Check sheet for the drawn part. Datum: minimum x, y, z corner. Units: mm. A direction names the side the tool comes from. Coordinates: 2 decimals unless noted, no trailing zeros. Order: outer loops, then holes, each group sorted by start corner. A loop starts at its lowest first (then second) coordinate and runs counter-clockwise, first axis right, second up. Notation, with made-up numbers: M -23,58.5 L -18,58.5 A13 cw -18,64.5 Z; hole C 85,-16 d7. An arc over 180 degrees is marked long. Return JSON: item names as keys, results as strings. Group by question number.
Q1. Section check A-A, the plane z = 24.5. Enter the section's corners in (x, y).
Q2. Section check C-C, the plane y = 24. Enter the section's corners in (x, z).
Q3. Mould release check, pull along Y, two halves, no side actions. Record for the marked faces 3, 4, 5 and 6: pulls with the +Y half, pulls with the -Y half, needs draft (parallel to the pull), parting line crosses it, or undercut.
Q4. Section check B-B, the plane x = 180. Enter the section's corners in (y, z), then the cut area to 3 significant figures.
Q5. Thickness scan on probe 1 along Y at (x, z) = (5, 22.5); probe 2 along X at (y, z) = (130.2, 18.25); probe 3 along X at (y, z) = (123.5, 24.75). Record the ranges inside material, lowest first.
Q6. Access from +Z, -Z, +X, -X, +Y, -Y to the whole of each face (thin tool, end or side, straight path). Record for the marked faces 1 and 2.
Q7. Section check D-D, the plane x = 37. Enter the section's corners in (y, z).
Q8. Go/stop test with flat-tipped pins: pin 1 Ø0.9 at (x, y) = (208.5, 5) entering from +Z; pin 2 Ø2.5 at (x, y) = (155.5, 89.5) entering from +Z. Record where each tip stops, or that it passes through.
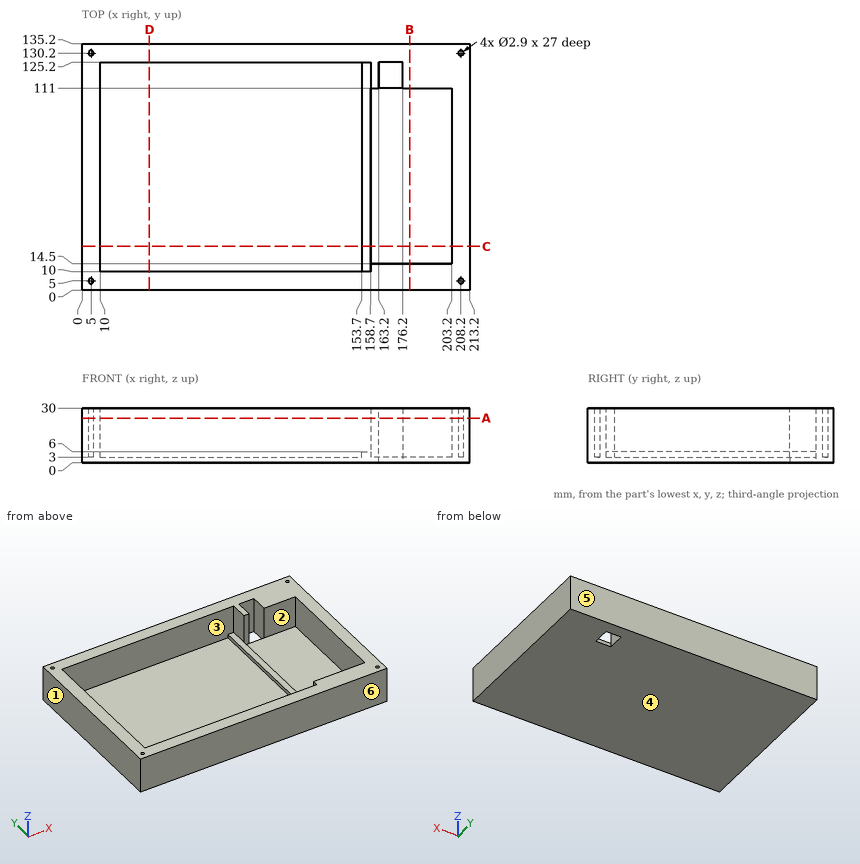
Numbers:
{
 "1": {"outline": "M 0,0 L 213.2,0 L 213.2,135.2 L 0,135.2 Z; hole C 5,5 d2.9; hole C 5,130.2 d2.9; hole M 10,10 L 158.7,10 L 158.7,14.5 L 203.2,14.5 L 203.2,111 L 176.2,111 L 176.2,125.2 L 163.2,125.2 L 163.2,111 L 158.7,111 L 158.7,125.2 L 10,125.2 Z; hole C 208.2,5 d2.9; hole C 208.2,130.2 d2.9"},
 "2": {"outline": "M 0,0 L 213.2,0 L 213.2,30 L 203.2,30 L 203.2,3 L 158.7,3 L 158.7,6 L 153.7,6 L 153.7,3 L 10,3 L 10,30 L 0,30 Z"},
 "3": {"face 3": "undercut", "face 4": "needs draft", "face 5": "pulls with the +Y half", "face 6": "pulls with the -Y half"},
 "4": {"outline": "M 0,0 L 135.2,0 L 135.2,30 L 111,30 L 111,3 L 14.5,3 L 14.5,30 L 0,30 Z", "area": "1,450 mm2"},
 "5": {"probe 1": "y = 0 to 3.55, 6.45 to 128.75, 131.65 to 135.2", "probe 2": "x = 0 to 3.55, 6.45 to 206.75, 209.65 to 213.2", "probe 3": "x = 0 to 10, 158.7 to 163.2, 176.2 to 213.2"},
 "6": {"face 1": "+Z, -Z, -X, +Y, -Y", "face 2": "+Z"},
 "7": {"outline": "M 0,0 L 135.2,0 L 135.2,30 L 125.2,30 L 125.2,3 L 10,3 L 10,30 L 0,30 Z"},
 "8": {"pin 1": "stops at z = 3", "pin 2": "stops at z = 6"}
}
